Can you work these out from the model? Positions are in its coordinate system, mm. Round coordinates to 2 decimals unless told otherwise and drop trailing zeros. Loops run counter-clockwise (first coordinate to the right, second up) from the corner with the lowest first, then second, coordinate; pieces in that order, holes last.
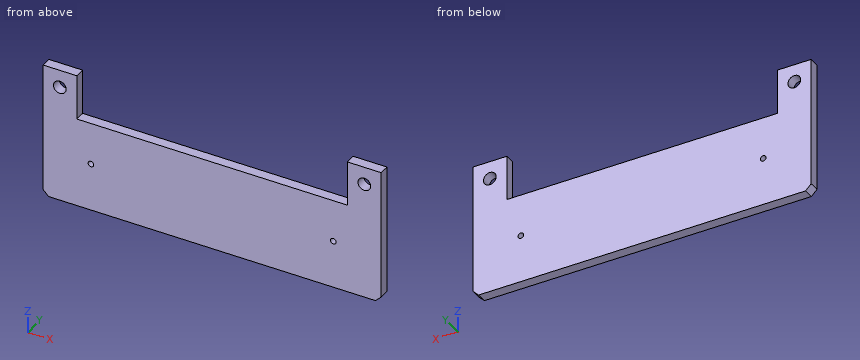
```python
from build123d import *

# Parameters (mm, degrees)
F0_R     = 2.5
F0_R_2   = 5.65
F1_DEPTH = 9


with BuildPart() as f1:
    # F0 (on Front) → F1 (new body)
    with BuildSketch(Plane.XZ):
        Polygon((-120, 120), (-150, 120), (-150, 5), (-145, 0), (0, 0), (145, 0), (150, 5), (150, 120), (120, 120), (120, 80), (0, 80), (-120, 80), align=None)
        with Locations((-107.5, 42.5)):
            Circle(F0_R, mode=Mode.SUBTRACT)
        with Locations((107.5, 42.5)):
            Circle(F0_R, mode=Mode.SUBTRACT)
        with Locations((-135.05, 104.35)):
            Circle(F0_R_2, mode=Mode.SUBTRACT)
        with Locations((135.05, 104.35)):
            Circle(F0_R_2, mode=Mode.SUBTRACT)
    extrude(amount=F1_DEPTH)


solid = f1.part
```
(1) Suppose I cut it at C-C (y = -4.25). Write out the boundary of the cut face in (x, z).
(2) Suppose I cut it at B-B (z = 104.35). Write out the boundary of the cut face in (x, y).
(3) Suppose I cut it at D-D (x = -32.5). Write out the boundary of the cut face in (y, z).
(4) If I drill on line 1 (X direction, y = -3.75, z = 91.5); line 2 (Z direction, x = 135.05, y = -2.75); line 3 (Z direction, x = -107.5, y = -4), over which ranges is the centre line in solid material (lowest first)?
(5) Suppose I cut it at A-A (x = 135.05). Write out the boundary of the cut face in (y, z), then the cut area to 3 significant figures.
(6) For pin 1 (1.5 mm diameter, centred on x = -0.5, y = -5, fed in from +Z), with a flat end and sliding along its axis, tell me the tip position at first contact or that it passes through.
Check result:
1. outline: (-150, 5) - (-145, 0) - (145, 0) - (150, 5) - (150, 120) - (120, 120) - (120, 80) - (-120, 80) - (-120, 120) - (-150, 120) - close; hole circle Ø11.3 at (-135.05, 104.35); hole circle Ø5 at (-107.5, 42.5); hole circle Ø5 at (107.5, 42.5); hole circle Ø11.3 at (135.05, 104.35)
2. outline: (-150, -9) - (-140.7, -9) - (-140.7, 0) - (-150, 0) - close; (-129.4, -9) - (-120, -9) - (-120, 0) - (-129.4, 0) - close; (120, -9) - (129.4, -9) - (129.4, 0) - (120, 0) - close; (140.7, -9) - (150, -9) - (150, 0) - (140.7, 0) - close
3. outline: (-9, 0) - (0, 0) - (0, 80) - (-9, 80) - close
4. line 1: x = -150 to -120, 120 to 150
4. line 2: z = 0 to 98.7, 110 to 120
4. line 3: z = 0 to 40, 45 to 80
5. outline: (-9, 0) - (0, 0) - (0, 98.7) - (-9, 98.7) - close; (-9, 110) - (0, 110) - (0, 120) - (-9, 120) - close
5. area: 978 mm2
6. pin 1: stops at z = 80
